The model under review builds one solid part; all positions refer to its coordinate system, in mm. Round coordinates to 2 decimals unless told otherwise and drop trailing zeros. Order: outer loops, then holes, each group sorted by start corner. A loop starts at its lowest first (then second) coordinate and runs counter-clockwise, first axis right, second up. Notation, with made-up numbers: M 65,-5.5 L 123,-5.5 A25 cw 123,33.5 Z; hole C 47,9.5 d1. An arc over 180 degrees is marked long. One line per item, written item: value. Start each with the question number.
from build123d import *

# Parameters (mm, degrees)
EXTRUDE1_DEPTH = 27.5


with BuildPart() as part:
    # Sketch1 → Extrude1 (new, symmetric)
    with BuildSketch(Plane.XY):
        with BuildLine():
            Line((-3.3, -2.4), (3.3, -2.4))
            Line((3.3, -2.4), (3.5, -2.2))
            Line((3.5, -2.2), (3.5, 0.106274607))
            ThreePointArc((3.5, 0.106274607), (3.091294745, 0.282570681), (2.840065792, 0.65))
            Line((2.840065792, 0.65), (2.340065792, 0.65))
            Line((2.340065792, 0.65), (2.340065792, 1.15))
            Line((2.340065792, 1.15), (2.840065792, 1.15))
            ThreePointArc((2.840065792, 1.15), (3.091294745, 1.517429319), (3.5, 1.693725393))
            Line((3.5, 1.693725393), (3.5, 2.2))
            Line((3.5, 2.2), (3.3, 2.4))
            Line((3.3, 2.4), (-3.3, 2.4))
            Line((-3.3, 2.4), (-3.5, 2.2))
            Line((-3.5, 2.2), (-3.5, 1.693725393))
            ThreePointArc((-3.5, 1.693725393), (-3.091294745, 1.517429319), (-2.840065792, 1.15))
            Line((-2.840065792, 1.15), (-2.340065792, 1.15))
            Line((-2.340065792, 1.15), (-2.340065792, 0.65))
            Line((-2.340065792, 0.65), (-2.840065792, 0.65))
            ThreePointArc((-2.840065792, 0.65), (-3.091294745, 0.282570681), (-3.5, 0.106274607))
            Line((-3.5, 0.106274607), (-3.5, -2.2))
            Line((-3.5, -2.2), (-3.3, -2.4))
        make_face()
    extrude(amount=EXTRUDE1_DEPTH, both=True)


solid = part.part
Item 1: Wall thickness on L1, parallel to Y at x = -2.5, z = 4; L2, parallel to X at y = 1.05, z = 3: over which ranges is each line inside the solid? List them lowest first.
Item 2: Clearance check with a flat-ended pin moving along its axis: P1, Ø1, axis at y = 1, z = 9, coming from the +X side. State where the tip first meets the part, or that it passes through.
Item 3: Consider section A-A, the plane z = 10. Give the boundary of the cut face in (x, y).
Computed:
1. L1: y = -2.4 to 0.65, 1.15 to 2.4
1. L2: x = -2.34 to 2.34
2. P1: stops at x = 3.07
3. outline: M -3.5,-2.2 L -3.3,-2.4 L 3.3,-2.4 L 3.5,-2.2 L 3.5,0.11 A0.8 cw 2.84,0.65 L 2.34,0.65 L 2.34,1.15 L 2.84,1.15 A0.8 cw 3.5,1.69 L 3.5,2.2 L 3.3,2.4 L -3.3,2.4 L -3.5,2.2 L -3.5,1.69 A0.8 cw -2.84,1.15 L -2.34,1.15 L -2.34,0.65 L -2.84,0.65 A0.8 cw -3.5,0.11 Z
